from build123d import *

# Parameters (mm, degrees)
BOSS_EXTRUDE1_DEPTH = 21.65
SKETCH1_3_R         = 5.75
BOSS_EXTRUDE2_DEPTH = 25.45
SKETCH1_4_R         = 2
BOSS_EXTRUDE3_DEPTH = 29.25
BOSS_EXTRUDE4_START = 16.3
BOSS_EXTRUDE4_DEPTH = 1.5


with BuildPart() as part:
    # Sketch1 → Boss-Extrude1 (new body)
    with BuildSketch(Plane(origin=(0, 0, 0), x_dir=(1, 0, 0), z_dir=(0, 1, 0))):
        Polygon((-10.9, -5.75), (10.9, -5.75), (11.9, -4.75), (11.9, 4.75), (10.9, 5.75), (-10.9, 5.75), (-11.9, 4.75), (-11.9, -4.75), align=None)
    extrude(amount=BOSS_EXTRUDE1_DEPTH)

    # Sketch1_3 → Boss-Extrude2 (add)
    with BuildSketch(Plane(origin=(0, 0, 0), x_dir=(1, 0, 0), z_dir=(0, 1, 0))):
        with Locations(Location((6.15, 0, 0), (0, 0, 270))):
            Circle(SKETCH1_3_R)
    extrude(amount=BOSS_EXTRUDE2_DEPTH)

    # Sketch1_4 → Boss-Extrude3 (add)
    with BuildSketch(Plane(origin=(0, 0, 0), x_dir=(1, 0, 0), z_dir=(0, 1, 0))):
        with Locations(Location((6.15, 0, 0), (0, 0, 270))):
            Circle(SKETCH1_4_R)
    extrude(amount=BOSS_EXTRUDE3_DEPTH)

    # Sketch1_5 → Boss-Extrude4 (add)
    with BuildSketch(Plane(origin=(0, 0, 0), x_dir=(1, 0, 0), z_dir=(0, 1, 0)).offset(BOSS_EXTRUDE4_START)):
        with BuildLine():
            Line((11.9, -4.75), (10.9, -5.75))
            Line((10.9, -5.75), (15.025, -5.75))
            Line((15.025, -5.75), (16.025, -4.75))
            Line((16.025, -4.75), (16.025, -0.6))
            Line((16.025, -0.6), (14.203746042, -0.979023774))
            ThreePointArc((14.203746042, -0.979023774), (13, 0), (14.203746042, 0.979023774))
            Line((14.203746042, 0.979023774), (16.025, 0.6))
            Line((16.025, 0.6), (16.025, 4.75))
            Line((16.025, 4.75), (15.025, 5.75))
            Line((15.025, 5.75), (10.9, 5.75))
            Line((10.9, 5.75), (11.9, 4.75))
            Line((11.9, 4.75), (11.9, 0))
            Line((11.9, 0), (11.9, -4.75))
        make_face()
        with BuildLine():
            Line((-15.025, -5.75), (-10.9, -5.75))
            Line((-10.9, -5.75), (-11.9, -4.75))
            Line((-11.9, -4.75), (-11.9, 0))
            Line((-11.9, 0), (-11.9, 4.75))
            Line((-11.9, 4.75), (-10.9, 5.75))
            Line((-10.9, 5.75), (-15.025, 5.75))
            Line((-15.025, 5.75), (-16.025, 4.75))
            Line((-16.025, 4.75), (-16.025, 0.6))
            Line((-16.025, 0.6), (-14.203746042, 0.979023774))
            ThreePointArc((-14.203746042, 0.979023774), (-13, 0), (-14.203746042, -0.979023774))
            Line((-14.203746042, -0.979023774), (-16.025, -0.6))
            Line((-16.025, -0.6), (-16.025, -4.75))
            Line((-16.025, -4.75), (-15.025, -5.75))
        make_face()
    extrude(amount=BOSS_EXTRUDE4_DEPTH)


solid = part.part
CAD build for the part. Positions are in the model's coordinates, mm. A direction names the side the tool comes from. Coordinates: 2 decimals unless noted, no trailing zeros. Loops run counter-clockwise (first coordinate to the right, second up) from the corner with the lowest first, then second, coordinate; pieces in that order, holes last. Notation, with made-up numbers: (12.5, -31) - (57.5, -31) arc R21 cw to (57.5, -26) - close; hole circle Ø1 at (43.25, 20.5). An arc over 180 degrees is marked (long way). Use one line per item in the form item = value. Start each with the question number.
1) Band-saw the part on A-A (y = 3). Give the cut face in (x, z).
2) Band-saw the part on B-B (z = 4.25). Give the cut face in (x, y) (3 decimals), and give its area (3 significant figures).
3) Drill centre lines: L1, parallel to Z at x = 14, y = 17.35; L2, parallel to Y at x = 9.5, z = 2; L3, parallel to Y at x = -12, z = 1.25. Where is each one in solid material? Low to high. Write a range as from..to.
4) Band-saw the part on C-C (x = 7.5). Give the cut face in (y, z).
5) Two-plate mould, pull along X, no slides. Class faces 6 (the face through (11, 21.65, -5)), 7 (the face through (16.025, 17, 3)), 8 (the face through (-15.127, 17.04, -0.787)): +X half, -X half, draft (parallel to the pull), parting line (faces both ways), or undercut.
6) Tool access for faces 1 (the face through (11, 21.65, 4)), 2 (the face through (-11.39, 8.04, -5.26)), 3 (the face through (-11.41, 19.7, 5.24)), 4 (the face through (0.537, 23.523, -1.246)), 5 (the face through (11.39, 8.04, 5.26)): list every direction of +Z, -Z, +X, -X, +Y, -Y with a clear straight run to the whole face (end or side of a thin tool).
7) Flat gauge pins, fed straight in: pin 1 (1.5 mm diameter, centred on y = 19.5, z = 4.5, fed in from +X); pin 2 (2 mm diameter, centred on y = 5, z = -2.5, fed in from -X); pin 3 (3 mm diameter, centred on x = 9.5, z = -4.5, fed in from +Y). Where does each tip first touch, or does it go through?
8) Band-saw the part on D-D (z = -2.5). Give the cut face in (x, y) (3 decimals), and give its area (3 significant figures).
Check values:
q1.outline = (-11.9, -4.75) - (-10.9, -5.75) - (10.9, -5.75) - (11.9, -4.75) - (11.9, 4.75) - (10.9, 5.75) - (-10.9, 5.75) - (-11.9, 4.75) - close
q2.outline = (-16.025, 16.3) - (-11.9, 16.3) - (-11.9, 0) - (11.9, 0) - (11.9, 16.3) - (16.025, 16.3) - (16.025, 17.8) - (11.9, 17.8) - (11.9, 21.65) - (10.023, 21.65) - (10.023, 25.45) - (2.277, 25.45) - (2.277, 21.65) - (-11.9, 21.65) - (-11.9, 17.8) - (-16.025, 17.8) - close
q2.area = 557 mm2
q3.L1 = -5.75..-1, 1..5.75
q3.L2 = 0..25.45
q3.L3 = 16.3..17.8
q4.outline = (0, -5.75) - (21.65, -5.75) - (21.65, -5.59) - (25.45, -5.59) - (25.45, -1.48) - (29.25, -1.48) - (29.25, 1.48) - (25.45, 1.48) - (25.45, 5.59) - (21.65, 5.59) - (21.65, 5.75) - (0, 5.75) - close
q5.face_6 = draft
q5.face_7 = +X half
q5.face_8 = undercut
q6.face_1 = +Z, +X, +Y
q6.face_2 = -Z, -X, -Y
q6.face_3 = +Z, -X, +Y
q6.face_4 = +Y
q6.face_5 = +Z, +X, -Y
q7.pin_1 = 11.9
q7.pin_2 = -11.9
q7.pin_3 = 25.45
q8.outline = (-16.025, 16.3) - (-11.9, 16.3) - (-11.9, 0) - (11.9, 0) - (11.9, 16.3) - (16.025, 16.3) - (16.025, 17.8) - (11.9, 17.8) - (11.9, 21.65) - (11.328, 21.65) - (11.328, 25.45) - (0.972, 25.45) - (0.972, 21.65) - (-11.9, 21.65) - (-11.9, 17.8) - (-16.025, 17.8) - close
q8.area = 567 mm2
